from build123d import *

# Parameters (mm, degrees)
F0_R     = 9
F0_R_2   = 7
F1_DEPTH = 7.5
F0_R_3   = 10.75
F2_DEPTH = 2.5
F3_SIZE  = 0.25
F4_R     = 2
F5_SIZE  = 1.2


with BuildPart() as f1:
    # F0 (on Top) → F1 (new body)
    with BuildSketch(Plane.XY):
        Circle(F0_R)
        Circle(F0_R_2, mode=Mode.SUBTRACT)
    extrude(amount=F1_DEPTH)

    # F0 (on Top) → F2 (join)
    with BuildSketch(Plane.XY):
        Circle(F0_R_3)
        Circle(F0_R, mode=Mode.SUBTRACT)
    extrude(amount=F2_DEPTH)

    # F3
    f3_edges = [f1.edges().sort_by_distance(p)[0] for p in [
        (-9, 0, 7.5),
        (-7, 0, 7.5),
    ]]
    chamfer(f3_edges, length=F3_SIZE)

    # F4
    f4_edges = [f1.edges().sort_by_distance(p)[0] for p in [
        (-10.75, 0, 0),
    ]]
    fillet(f4_edges, radius=F4_R)

    # F5
    f5_edges = [f1.edges().sort_by_distance(p)[0] for p in [
        (-7, 0, 0),
    ]]
    chamfer(f5_edges, length=F5_SIZE)


solid = f1.part
Here's how the part is built. I have some questions about the finished solid (model axes, mm). A direction names the side the tool comes from. Round coordinates to 2 decimals unless told otherwise and drop trailing zeros. Order: outer loops, then holes, each group sorted by start corner. A loop starts at its lowest first (then second) coordinate and runs counter-clockwise, first axis right, second up. Notation, with made-up numbers: (79.25, -18.75) -> (121.25, -18.75) arc R17 cw to (121.25, 11.25) -> close; hole circle Ø1 at (58, 31). An arc over 180 degrees is marked (long way). Return JSON: item names as keys, results as strings.
Q1. If we mould it in two halves opening along Y, with no side actions, what happens to faces 3 (the flat face through (-8, -3, 0)), 4 (the cylindrical face through (6.466, -2.681, 4.183)), 5 (the cylindrical face through (-1.4, 10.66, 2.25))? For each: released by +Y, released by -Y, zero draft, split by the parting line, or undercut.
Filled sheet:
{"face 3": "zero draft", "face 4": "undercut", "face 5": "split by the parting line"}
Q2. If we section it at C-C on z = 4.5: List the corners of the cut face in (x, y) for me.
Filled sheet:
{"outline": "circle Ø18 at (0, 0); hole circle Ø14 at (0, 0)"}
Q3. For pin 1 Ø2 at (x, y) = (1, 6.5) entering from -Z; pin 2 Ø2 at (x, z) = (3, 4) entering from -Y, each with a flat end and sliding along its axis, tell me the tip position at first contact or that it passes through.
Filled sheet:
{"pin 1": "stops at z = 0.62", "pin 2": "stops at y = -8.77"}
Q4. Which directions (+Z, -Z, +X, -X, +Y, -Y) give clear straight access to the entire face, cutting with the end or side of a thin tool? Please do faces 1 (the flat face through (-3, 7, 7.5)), 2 (the flat face through (-2, -9, 2.5)).
Filled sheet:
{"face 1": "+Z, +X, -X, +Y, -Y", "face 2": "+Z"}
Q5. If we section it at A-A on x = 0: List the corners of the cut face in (y, z) for me.
Filled sheet:
{"outline": "(-10.75, 2) arc R2 ccw to (-8.75, 0) -> (-8.2, 0) -> (-7, 1.2) -> (-7, 7.25) -> (-7.25, 7.5) -> (-8.75, 7.5) -> (-9, 7.25) -> (-9, 2.5) -> (-10.75, 2.5) -> close; (7, 1.2) -> (8.2, 0) -> (8.75, 0) arc R2 ccw to (10.75, 2) -> (10.75, 2.5) -> (9, 2.5) -> (9, 7.25) -> (8.75, 7.5) -> (7.25, 7.5) -> (7, 7.25) -> close"}
Q6. I need wall thicknesses on line 1 along Y through (x, z) = (0, 6.25); line 2 along Y through (x, z) = (-1.5, 1.75); line 3 along X through (y, z) = (3, 5). Which ranges of each line are inside material? Lowest first, please. Write a range as from..to.
Filled sheet:
{"line 1": "y = -9..-7, 7..9", "line 2": "y = -10.63..-6.84, 6.84..10.63", "line 3": "x = -8.49..-6.32, 6.32..8.49"}
